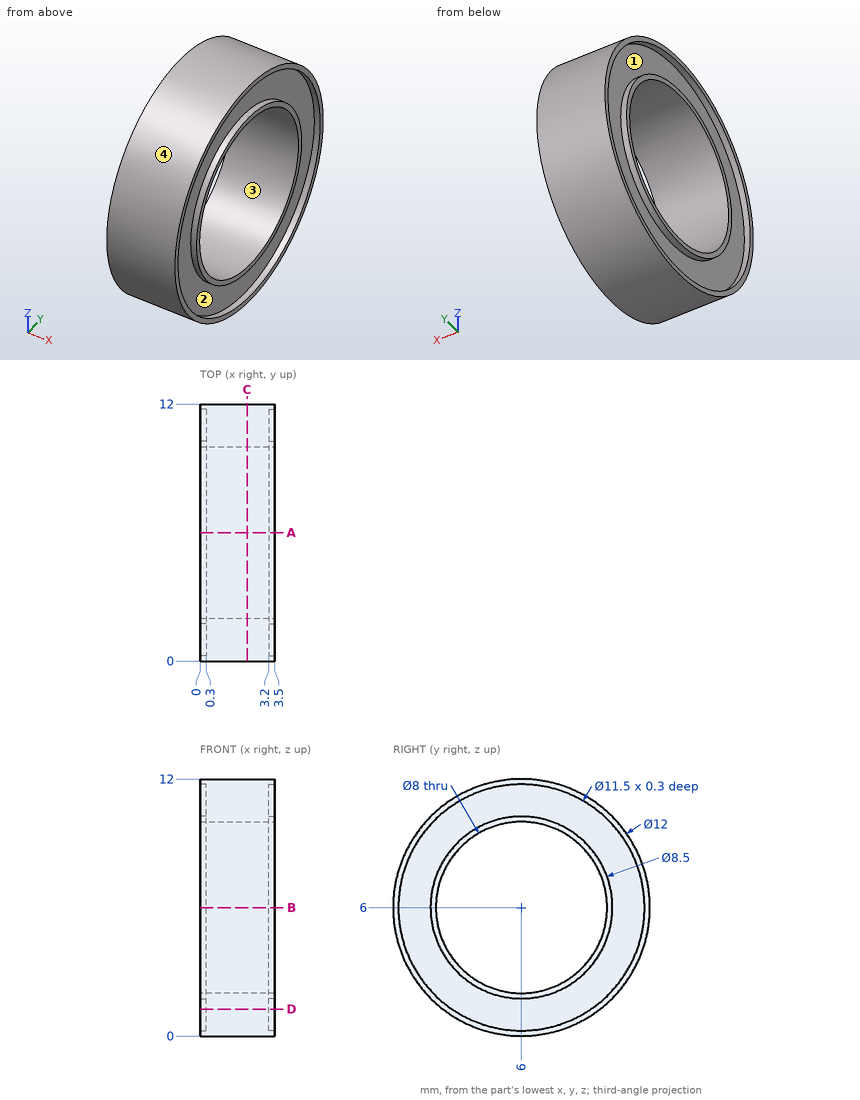
Design review of the part shown in the three views and the two pictorial views. Dimensions are in mm from the part's minimum x, y and z. A direction names the side the tool comes from. Round coordinates to 2 decimals unless told otherwise and drop trailing zeros. Write each loop counter-clockwise with the first axis right and the second up, starting at its lowest first coordinate (ties: lowest second). Pieces come first, ordered by that corner, then holes. Notation, with made-up numbers: (-28, 81) - (-8, 81) arc R26 ccw to (-8, 111) - close; hole circle Ø8 at (21, 32). An arc over 180 degrees is marked (long way). Answer as CSV lines item,"result". Start each with the question number.
(1) For pin 1 (5 mm diameter, centred on y = 6, z = 6, fed in from -X); pin 2 (6 mm diameter, centred on y = 6.5, z = 4.5, fed in from +X); pin 3 (1 mm diameter, centred on x = 2, z = 2.5, fed in from +Y); pin 4 (1 mm diameter, centred on x = 3, z = 8, fed in from -Y), all flat-tipped, find the tip position at first contact; note any pin that passes through.
(2) Add section D-D, the plane z = 1.25. State the section outline as (x, y) points, plus the area to 3 significant figures.
(3) Add section C-C, the plane x = 2.2. State the section outline as (y, z) points, plus the area to 3 significant figures.
(4) For line 1 (Y direction, x = 0.1, z = 6); line 2 (Y direction, x = 2.7, z = 6); line 3 (X direction, y = 2.75, z = 10), list the stretches that pass through material, from the lowest coordinate up.
(5) Add section A-A, the plane y = 6. State the section outline as (x, z) points.
(6) Machinability: for the marked faces 1 and 2, which of the approach directions +Z, -Z, +X, -X, +Y, -Y give a long, thin tool a straight path to every point of the face, cutting with its end or side? Answer none if there is none.
(7) Mouldability with a two-part tool opening along Z and no side actions: class the marked faces 3 and 4 as +Z half, -Z half, draft (parallel to the pull), parting line (faces both ways), or undercut.
From the geometry:
1,pin 1,"passes through"
1,pin 2,"stops at x = 3.5"
1,pin 3,"stops at y = 11.2"
1,pin 4,"stops at y = 0.19"
2,outline,"(0, 2.33) - (3.5, 2.33) - (3.5, 2.76) - (3.2, 2.76) - (3.2, 9.24) - (3.5, 9.24) - (3.5, 9.67) - (0, 9.67) - (0, 9.24) - (0.3, 9.24) - (0.3, 2.76) - (0, 2.76) - close"
2,area,"21.8 mm²"
3,outline,"circle Ø12 at (6, 6); hole circle Ø8 at (6, 6)"
3,area,"62.8 mm²"
4,line 1,"y = 0 to 0.25, 1.75 to 2, 10 to 10.25, 11.75 to 12"
4,line 2,"y = 0 to 2, 10 to 12"
4,line 3,"x = 0.3 to 3.2"
5,outline,"(0, 0) - (3.5, 0) - (3.5, 0.25) - (3.2, 0.25) - (3.2, 1.75) - (3.5, 1.75) - (3.5, 2) - (0, 2) - (0, 1.75) - (0.3, 1.75) - (0.3, 0.25) - (0, 0.25) - close; (0, 10) - (3.5, 10) - (3.5, 10.25) - (3.2, 10.25) - (3.2, 11.75) - (3.5, 11.75) - (3.5, 12) - (0, 12) - (0, 11.75) - (0.3, 11.75) - (0.3, 10.25) - (0, 10.25) - close"
6,face 1,"-X"
6,face 2,"+X"
7,face 3,"undercut"
7,face 4,"parting line"
